For this review, take the finished solid that the model builds, in its own axes (mm). Face numbers are marked on the shaded views. A direction names the side the tool comes from. Coordinates: 2 decimals unless noted, no trailing zeros. Write each loop counter-clockwise with the first axis right and the second up, starting at its lowest first coordinate (ties: lowest second). Pieces come first, ordered by that corner, then holes.
1) For the marked faces 1 and 2, list the 3-axis set-ups (+Z, -Z, +X, -X, +Y, -Y) from which the entire face can be reached by the end or side of a thin tool; tool diameter is ignored.
2) Insertion check: P1, Ø5, axis at y = -2, z = 9, coming from the -X side; P2, Ø2, axis at x = 8, y = -8.5, coming from the +Z side; P3, Ø5, axis at y = -5.5, z = 18, coming from the +X side; P4, Ø6, axis at x = 17.79, y = -5, coming from the +Z side. Each pin has a flat end and moves straight along its axis. Give the tip position at first contact, or say it passes through.
3) Mouldability with a two-part tool opening along Y and no side actions: class the marked faces 3, 4, 5 and 6 as pulls with the +Y half, pulls with the -Y half, needs draft (parallel to the pull), parting line crosses it, or undercut.
4) To check wall thickness, follow line 1 along Y through (x, z) = (1, 19); line 2 along X through (y, z) = (-1, 13.75); line 3 along Z through (x, y) = (0, -7). State the ranges of each line that lie inside material, in increasing order.
5) We need section C-C on z = 13.75. Write out the cut boundary in (x, y).
6) We need section B-B on x = 14.25. Write out the cut boundary in (y, z).
7) We need section A-A on y = -5. Give the number of separate pieces and of enclosed holes in the cut face, then the cut area to 3 significant figures.
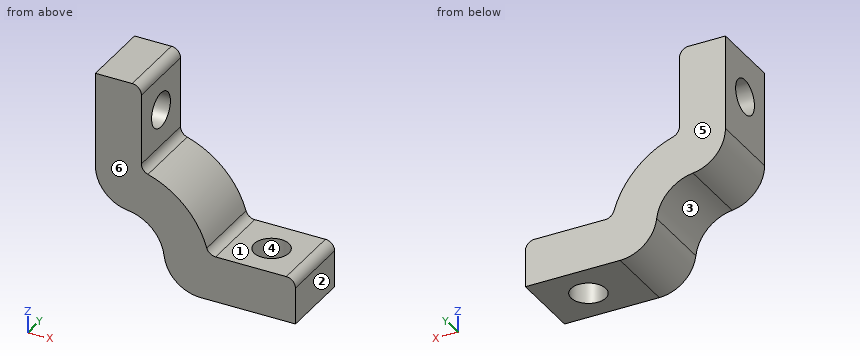
from build123d import *

# Parameters (mm, degrees)
F1_DEPTH = 10
F2_R     = 2.4
F3_DEPTH = 6.35
F7_R     = 5.08
F8_R     = 1.27


# Not quite as in the source:
# - a pattern or mirror of a feature is missing from the dataset's text; its kind, count and spacing are read off the source's solid


with BuildPart() as f1:
    # F0 (on Front) → F1 (new body)
    with BuildSketch(Plane.XZ):
        with BuildLine():
            ThreePointArc((0, 5.715), (4.0411152545, 4.0411152545), (5.715, 0))
            Line((5.715, 0), (5.715, -3.81))
            Line((5.715, -3.81), (23.7946015193, -3.81))
            Line((23.7946015193, -3.81), (23.7946015193, 2.54))
            Line((23.7946015193, 2.54), (11.7946015193, 2.54))
            ThreePointArc((11.7946015193, 2.54), (8.531243315, 8.531243315), (2.54, 11.7946015193))
            Line((2.54, 11.7946015193), (2.54, 23.7946015193))
            Line((2.54, 23.7946015193), (-3.81, 23.7946015193))
            Line((-3.81, 23.7946015193), (-3.81, 5.715))
            Line((-3.81, 5.715), (0, 5.715))
        make_face()
    extrude(amount=F1_DEPTH)

    # F2 (on face) → F3 (cut, through all)
    with BuildSketch(Plane.XY.offset(2.54)):
        with Locations((17.7946015193, -5)):
            Circle(F2_R)
    f3 = extrude(amount=-F3_DEPTH, mode=Mode.SUBTRACT)

    # F3_copies: F3 across plane
    add(f3.mirror(Plane(origin=(0, 0, 0), x_dir=(0.7071067812, 0, 0.7071067812), z_dir=(-0.7071067812, 0, 0.7071067812))), mode=Mode.SUBTRACT)

    # F7
    f7_edges = [f1.edges().sort_by_distance(p)[0] for p in [
        (-3.81, -5, 5.715),
        (5.715, -5, -3.81),
    ]]
    fillet(f7_edges, radius=F7_R)

    # F8
    f8_edges = [f1.edges().sort_by_distance(p)[0] for p in [
        (2.54, -5, 23.794602),
        (2.54, -5, 11.794602),
        (11.794602, -5, 2.54),
        (23.794602, -5, 2.54),
    ]]
    fillet(f8_edges, radius=F8_R)


solid = f1.part
Result:
1. face 1: +Z, +X, +Y, -Y
1. face 2: +Z, -Z, +X, +Y, -Y
2. P1: stops at x = -3.81
2. P2: stops at z = 9.83
2. P3: stops at x = 2.54
2. P4: stops at z = 2.54
3. face 3: needs draft
3. face 4: undercut
3. face 5: pulls with the +Y half
3. face 6: pulls with the -Y half
4. line 1: y = -10 to -7.08, -2.92 to 0
4. line 2: x = -3.81 to 2.54
4. line 3: z = 5.8 to 16.47, 19.12 to 23.79
5. outline: (-3.81, -10) - (2.54, -10) - (2.54, 0) - (-3.81, 0) - close
6. outline: (-10, -3.81) - (0, -3.81) - (0, 2.54) - (-10, 2.54) - close
7. separate pieces: 3
7. enclosed holes: 0
7. area: 215 mm2
